```python
from build123d import *

# Parameters (mm, degrees)
BOSS_EXTRUDE1_DEPTH = 3.6
BOSS_EXTRUDE2_DEPTH = 1.5
CUT_EXTRUDE1_DEPTH  = 3.6
BOSS_EXTRUDE5_DEPTH = 3.6
CHAMFER1_SIZE       = 3.6
CHAMFER1_SIZE_2     = 0.062838234
FILLET3_R           = 1
FILLET4_R           = 0.5


with BuildPart() as part:
    # Sketch1 → Boss-Extrude1 (new body)
    with BuildSketch(Plane(origin=(0, 0, 0), x_dir=(1, 0, 0), z_dir=(0, 1, 0))):
        with BuildLine():
            Line((6, 0), (26.9, 0))
            ThreePointArc((26.9, 0), (31.142640687, 1.757359313), (32.9, 6))
            Line((32.9, 6), (32.9, 17.9))
            ThreePointArc((32.9, 17.9), (31.142640687, 22.142640687), (26.9, 23.9))
            Line((26.9, 23.9), (6, 23.9))
            ThreePointArc((6, 23.9), (1.757359313, 22.142640687), (0, 17.9))
            Line((0, 17.9), (0, 6))
            ThreePointArc((0, 6), (1.757359313, 1.757359313), (6, 0))
        make_face()
    extrude(amount=BOSS_EXTRUDE1_DEPTH)

    # Sketch2 → Boss-Extrude2 (add)
    with BuildSketch(Plane(origin=(0, 3.6, 0), x_dir=(1, 0, 0), z_dir=(0, 1, 0))):
        with BuildLine():
            Line((4.75, 25.15), (28.15, 25.15))
            ThreePointArc((28.15, 25.15), (33.099747468, 23.099747468), (35.15, 18.15))
            Line((35.15, 18.15), (35.15, 4.75))
            ThreePointArc((35.15, 4.75), (33.099747468, -0.199747468), (28.15, -2.25))
            Line((28.15, -2.25), (4.75, -2.25))
            ThreePointArc((4.75, -2.25), (-0.199747468, -0.199747468), (-2.25, 4.75))
            Line((-2.25, 4.75), (-2.25, 18.15))
            ThreePointArc((-2.25, 18.15), (-0.199747468, 23.099747468), (4.75, 25.15))
        make_face()
    extrude(amount=BOSS_EXTRUDE2_DEPTH)

    # Sketch3 → Cut-Extrude1 (cut)
    with BuildSketch(Plane.XZ):
        with BuildLine():
            Line((25.7, -22.7), (7.2, -22.7))
            ThreePointArc((7.2, -22.7), (2.957359313, -20.942640687), (1.2, -16.7))
            Line((1.2, -16.7), (1.2, -7.2))
            ThreePointArc((1.2, -7.2), (2.957359313, -2.957359313), (7.2, -1.2))
            Line((7.2, -1.2), (25.7, -1.2))
            ThreePointArc((25.7, -1.2), (29.942640687, -2.957359313), (31.7, -7.2))
            Line((31.7, -7.2), (31.7, -16.7))
            ThreePointArc((31.7, -16.7), (29.942640687, -20.942640687), (25.7, -22.7))
        make_face()
    extrude(amount=-CUT_EXTRUDE1_DEPTH, mode=Mode.SUBTRACT)

    # Sketch5 → Boss-Extrude5 (add)
    with BuildSketch(Plane.XZ.offset(-3.6)):
        with BuildLine():
            Line((7.2, -1.2), (8.4, -1.2))
            Line((8.4, -1.2), (8.4, -6.2))
            ThreePointArc((8.4, -6.2), (8.692893219, -6.907106781), (9.4, -7.2))
            Line((9.4, -7.2), (23.5, -7.2))
            ThreePointArc((23.5, -7.2), (24.207106781, -6.907106781), (24.5, -6.2))
            Line((24.5, -6.2), (24.5, -1.2))
            Line((24.5, -1.2), (25.7, -1.2))
            Line((25.7, -1.2), (25.7, -6.2))
            ThreePointArc((25.7, -6.2), (25.992893219, -6.907106781), (26.7, -7.2))
            Line((26.7, -7.2), (31.7, -7.2))
            Line((31.7, -7.2), (31.7, -8.4))
            Line((31.7, -8.4), (26.7, -8.4))
            ThreePointArc((26.7, -8.4), (25.992893219, -8.692893219), (25.7, -9.4))
            Line((25.7, -9.4), (25.7, -14.5))
            ThreePointArc((25.7, -14.5), (25.992893219, -15.207106781), (26.7, -15.5))
            Line((26.7, -15.5), (31.7, -15.5))
            Line((31.7, -15.5), (31.7, -16.7))
            Line((31.7, -16.7), (26.7, -16.7))
            ThreePointArc((26.7, -16.7), (25.992893219, -16.992893219), (25.7, -17.7))
            Line((25.7, -17.7), (25.7, -22.7))
            Line((25.7, -22.7), (24.5, -22.7))
            Line((24.5, -22.7), (24.5, -17.7))
            ThreePointArc((24.5, -17.7), (24.207106781, -16.992893219), (23.5, -16.7))
            Line((23.5, -16.7), (9.4, -16.7))
            ThreePointArc((9.4, -16.7), (8.692893219, -16.992893219), (8.4, -17.7))
            Line((8.4, -17.7), (8.4, -22.7))
            Line((8.4, -22.7), (7.2, -22.7))
            Line((7.2, -22.7), (7.2, -17.7))
            ThreePointArc((7.2, -17.7), (6.907106781, -16.992893219), (6.2, -16.7))
            Line((6.2, -16.7), (1.2, -16.7))
            Line((1.2, -16.7), (1.2, -15.5))
            Line((1.2, -15.5), (6.2, -15.5))
            ThreePointArc((6.2, -15.5), (6.907106781, -15.207106781), (7.2, -14.5))
            Line((7.2, -14.5), (7.2, -9.4))
            ThreePointArc((7.2, -9.4), (6.907106781, -8.692893219), (6.2, -8.4))
            Line((6.2, -8.4), (1.2, -8.4))
            Line((1.2, -8.4), (1.2, -7.2))
            Line((1.2, -7.2), (6.2, -7.2))
            ThreePointArc((6.2, -7.2), (6.907106781, -6.907106781), (7.2, -6.2))
            Line((7.2, -6.2), (7.2, -1.2))
        make_face()
        with BuildLine():
            Line((9.4, -8.4), (23.5, -8.4))
            ThreePointArc((23.5, -8.4), (24.207106781, -8.692893219), (24.5, -9.4))
            Line((24.5, -9.4), (24.5, -14.5))
            ThreePointArc((24.5, -14.5), (24.207106781, -15.207106781), (23.5, -15.5))
            Line((23.5, -15.5), (9.4, -15.5))
            ThreePointArc((9.4, -15.5), (8.692893219, -15.207106781), (8.4, -14.5))
            Line((8.4, -14.5), (8.4, -9.4))
            ThreePointArc((8.4, -9.4), (8.692893219, -8.692893219), (9.4, -8.4))
        make_face(mode=Mode.SUBTRACT)
    extrude(amount=BOSS_EXTRUDE5_DEPTH)

    # Chamfer1
    # the kernel refuses this chamfer: 3.6, 0.062838234 mm, written as the material it takes off along each edge
    with BuildSketch(Plane(origin=(0, 0, -17.9), x_dir=(-0.0006712501823120534, 0.9999997747115711, 0), z_dir=(0, 0, 1))) as chamfer1_piece_1_section:
        Polygon((CHAMFER1_SIZE * 0.999999774712, -CHAMFER1_SIZE * 0.000671250182312), (-CHAMFER1_SIZE_2 * 0.000671250179552, -CHAMFER1_SIZE_2 * 0.999999770599), (0, 0), align=None)
    chamfer1_piece_1 = extrude(amount=11.9, mode=Mode.PRIVATE)
    chamfer1_piece_1 = split(chamfer1_piece_1, bisect_by=Plane(origin=(-0.01902042, 3.6, -11.95), z_dir=(0, -1, 0)), keep=Keep.TOP, mode=Mode.PRIVATE)
    add(chamfer1_piece_1, mode=Mode.SUBTRACT)
    with BuildSketch(Plane(origin=(6, 0, -6), x_dir=(-1, 0, 0), z_dir=(0, 0, -1))) as chamfer1_piece_2_section:
        Polygon((6, CHAMFER1_SIZE), (6 - CHAMFER1_SIZE_2 * 0.999999995888, 0), (6, 0), align=None)
    chamfer1_piece_2 = revolve(axis=Axis((6, 0, -6), (0, 1, 0)), revolution_arc=90, mode=Mode.PRIVATE)
    chamfer1_piece_2 = split(chamfer1_piece_2, bisect_by=Plane(origin=(1.769655981, 3.6, -1.769655981), z_dir=(0, -1, 0)), keep=Keep.TOP, mode=Mode.PRIVATE)
    add(chamfer1_piece_2, mode=Mode.SUBTRACT)
    with BuildSketch(Plane(origin=(6, 0, -17.9), x_dir=(0, 0, -1), z_dir=(1, 0, 0))) as chamfer1_piece_3_section:
        Polygon((6, CHAMFER1_SIZE), (6 - CHAMFER1_SIZE_2 * 0.999999995888, 0), (6, 0), align=None)
    chamfer1_piece_3 = revolve(axis=Axis((6, 0, -17.9), (0, 1, 0)), revolution_arc=90, mode=Mode.PRIVATE)
    chamfer1_piece_3 = split(chamfer1_piece_3, bisect_by=Plane(origin=(1.769655981, 3.6, -22.130344019), z_dir=(0, -1, 0)), keep=Keep.TOP, mode=Mode.PRIVATE)
    add(chamfer1_piece_3, mode=Mode.SUBTRACT)
    with BuildSketch(Plane(origin=(6, 0, 0), x_dir=(0, 0.9999997747115711, 0.0006712501823120534), z_dir=(1, 0, 0))) as chamfer1_piece_4_section:
        Polygon((CHAMFER1_SIZE * 0.999999774712, -CHAMFER1_SIZE * 0.000671250182312), (-CHAMFER1_SIZE_2 * 0.000671250179552, -CHAMFER1_SIZE_2 * 0.999999770599), (0, 0), align=None)
    chamfer1_piece_4 = extrude(amount=20.9, mode=Mode.PRIVATE)
    chamfer1_piece_4 = split(chamfer1_piece_4, bisect_by=Plane(origin=(16.45, 3.6, 0.01902042), z_dir=(0, -1, 0)), keep=Keep.TOP, mode=Mode.PRIVATE)
    add(chamfer1_piece_4, mode=Mode.SUBTRACT)
    with BuildSketch(Plane(origin=(26.9, 0, -23.9), x_dir=(0, 0.9999997747115711, -0.0006712501823119971), z_dir=(-1, 0, 0))) as chamfer1_piece_5_section:
        Polygon((CHAMFER1_SIZE * 0.999999774712, -CHAMFER1_SIZE * 0.000671250182312), (-CHAMFER1_SIZE_2 * 0.000671250179552, -CHAMFER1_SIZE_2 * 0.999999770599), (0, 0), align=None)
    chamfer1_piece_5 = extrude(amount=20.9, mode=Mode.PRIVATE)
    chamfer1_piece_5 = split(chamfer1_piece_5, bisect_by=Plane(origin=(16.45, 3.6, -23.91902042), z_dir=(0, -1, 0)), keep=Keep.TOP, mode=Mode.PRIVATE)
    add(chamfer1_piece_5, mode=Mode.SUBTRACT)
    with BuildSketch(Plane(origin=(26.9, 0, -6), x_dir=(0, 0, 1), z_dir=(-1, 0, 0))) as chamfer1_piece_6_section:
        Polygon((6, CHAMFER1_SIZE), (6 - CHAMFER1_SIZE_2 * 0.999999995888, 0), (6, 0), align=None)
    chamfer1_piece_6 = revolve(axis=Axis((26.9, 0, -6), (0, 1, 0)), revolution_arc=90, mode=Mode.PRIVATE)
    chamfer1_piece_6 = split(chamfer1_piece_6, bisect_by=Plane(origin=(31.130344019, 3.6, -1.769655981), z_dir=(0, -1, 0)), keep=Keep.TOP, mode=Mode.PRIVATE)
    add(chamfer1_piece_6, mode=Mode.SUBTRACT)
    with BuildSketch(Plane(origin=(26.9, 0, -17.9), x_dir=(1, 0, 0), z_dir=(0, 0, 1))) as chamfer1_piece_7_section:
        Polygon((6, CHAMFER1_SIZE), (6 - CHAMFER1_SIZE_2 * 0.999999995888, 0), (6, 0), align=None)
    chamfer1_piece_7 = revolve(axis=Axis((26.9, 0, -17.9), (0, 1, 0)), revolution_arc=90, mode=Mode.PRIVATE)
    chamfer1_piece_7 = split(chamfer1_piece_7, bisect_by=Plane(origin=(31.130344019, 3.6, -22.130344019), z_dir=(0, -1, 0)), keep=Keep.TOP, mode=Mode.PRIVATE)
    add(chamfer1_piece_7, mode=Mode.SUBTRACT)
    with BuildSketch(Plane(origin=(32.9, 0, -6), x_dir=(0.000671250182312946, 0.9999997747115711, 0), z_dir=(0, 0, -1))) as chamfer1_piece_8_section:
        Polygon((CHAMFER1_SIZE * 0.999999774712, -CHAMFER1_SIZE * 0.000671250182313), (-CHAMFER1_SIZE_2 * 0.000671250179553, -CHAMFER1_SIZE_2 * 0.999999770599), (0, 0), align=None)
    chamfer1_piece_8 = extrude(amount=11.9, mode=Mode.PRIVATE)
    chamfer1_piece_8 = split(chamfer1_piece_8, bisect_by=Plane(origin=(32.91902042, 3.6, -11.95), z_dir=(0, -1, 0)), keep=Keep.TOP, mode=Mode.PRIVATE)
    add(chamfer1_piece_8, mode=Mode.SUBTRACT)

    # Fillet3
    fillet3_edges = [part.edges().sort_by_distance(p)[0] for p in [
        (1.2, 1.8, -8.4),
        (1.2, 1.8, -15.5),
        (8.4, 1.8, -22.7),
        (24.5, 1.8, -22.7),
        (31.7, 1.8, -15.5),
        (31.7, 1.8, -8.4),
        (24.5, 1.8, -1.2),
        (8.4, 1.8, -1.2),
        (7.2, 1.8, -22.7),
        (1.2, 1.8, -16.7),
        (1.2, 1.8, -7.2),
        (7.2, 1.8, -1.2),
        (25.7, 1.8, -1.2),
        (31.7, 1.8, -7.2),
        (31.7, 1.8, -16.7),
        (25.7, 1.8, -22.7),
    ]]
    fillet(fillet3_edges, radius=FILLET3_R)

    # Fillet4
    fillet4_edges = [part.edges().sort_by_distance(p)[0] for p in [
        (-0.199747468, 5.1, 0.199747468),
        (16.45, 5.1, 2.25),
        (33.099747468, 5.1, 0.199747468),
        (35.15, 5.1, -11.45),
        (33.099747468, 5.1, -23.099747468),
        (16.45, 5.1, -25.15),
        (-0.199747468, 5.1, -23.099747468),
        (-2.25, 5.1, -11.45),
    ]]
    fillet(fillet4_edges, radius=FILLET4_R)


solid = part.part
```
Geometry check sheet. Reference: the model listing, model coordinates, mm. A direction names the side the tool comes from. Round coordinates to 2 decimals unless told otherwise and drop trailing zeros. Loops run counter-clockwise (first coordinate to the right, second up) from the corner with the lowest first, then second, coordinate; pieces in that order, holes last. Notation, with made-up numbers: (73, -1.5) - (131, -1.5) arc R30 ccw to (131, 35.5) - close; hole circle Ø9 at (-32.75, 84.5). An arc over 180 degrees is marked (long way). Use a Markdown table: item, result.
Q1. Material ranges on line 1 (X direction, y = 0.3, z = -14.5); line 2 (Z direction, x = 27, y = 2.4); line 3 (X direction, y = 2.5, z = -8.75), recorded low to high.
Solutions:
| item | result |
|---|---|
| line 1 | x = 0.06 to 1.2, 7.2 to 8.4, 24.5 to 25.7, 31.7 to 32.84 |
| line 2 | z = -23.88 to -22.56, -16.7 to -15.5, -8.4 to -7.2, -1.34 to -0.02 |
| line 3 | x = 0.02 to 1.44, 6.96 to 8.64, 24.26 to 25.94, 31.46 to 32.88 |
Q2. Go/stop test with flat-tipped pins: P1, Ø3, axis at x = 17, y = 2, coming from the -Z side; P2, Ø3, axis at x = 27.5, z = -19, coming from the -Y side; P3, Ø1.8, axis at x = 3.5, y = 1.5, coming from the -Z side; P4, Ø6.5, axis at x = 5.5, z = -5, coming from the -Y side. Record where each tip stops, or that it passes through.
Solutions:
| item | result |
|---|---|
| P1 | stops at z = -23.9 |
| P2 | stops at y = 3.6 |
| P3 | stops at z = -23.65 |
| P4 | stops at y = 0 |
Q3. Cross-section at B-B on z = -10. Record the cut outline in (x, y).
Solutions:
| item | result |
|---|---|
| outline | (-2.25, 3.6) - (0, 3.6) - (0.06, 0) - (1.2, 0) - (1.2, 3.6) - (7.2, 3.6) - (7.2, 0) - (8.4, 0) - (8.4, 3.6) - (24.5, 3.6) - (24.5, 0) - (25.7, 0) - (25.7, 3.6) - (31.7, 3.6) - (31.7, 0) - (32.84, 0) - (32.9, 3.6) - (35.15, 3.6) - (35.15, 4.6) arc R0.5 ccw to (34.65, 5.1) - (-1.75, 5.1) arc R0.5 ccw to (-2.25, 4.6) - close |
Q4. Draft check along X on faces 3 (the flat face through (17, 5.1, -12)), 4 (the flat face through (35.15, 4, -12)), 5 (the flat face through (16, 2, -8.4)). Enter one of: released by +X, released by -X, zero draft, split by the parting line, or undercut.
Solutions:
| item | result |
|---|---|
| face 3 | zero draft |
| face 4 | released by +X |
| face 5 | undercut |
Q5. Cross-section at A-A on x = 14. Record the cut outline in (y, z), plus the area to 3 significant figures.
Solutions:
| item | result |
|---|---|
| outline | (0, -23.84) - (3.6, -23.9) - (3.6, -25.15) - (4.6, -25.15) arc R0.5 ccw to (5.1, -24.65) - (5.1, 1.75) arc R0.5 ccw to (4.6, 2.25) - (3.6, 2.25) - (3.6, 0) - (0, -0.06) - (0, -1.2) - (3.6, -1.2) - (3.6, -7.2) - (0, -7.2) - (0, -8.4) - (3.6, -8.4) - (3.6, -15.5) - (0, -15.5) - (0, -16.7) - (3.6, -16.7) - (3.6, -22.7) - (0, -22.7) - close |
| area | 58.0 mm2 |
Q6. Cross-section at D-D on y = 0.5. State how many separate pieces and enclosed holes the cut face has, plus the area to 3 significant figures.
Solutions:
| item | result |
|---|---|
| separate pieces | 1 |
| enclosed holes | 9 |
| area | 251 mm2 |
Q7. Access from +Z, -Z, +X, -X, +Y, -Y to the whole of each face (thin tool, end or side, straight path). Record for faces 1 (the cylindrical face through (33, 4.1, -23.2)), 2 (the flat face through (7.2, 2, -4)).
Solutions:
| item | result |
|---|---|
| face 1 | -Z, +X, +Y, -Y |
| face 2 | -Y |
Q8. Cross-section at C-C on y = 4.15. Record the cut outline in (x, z).
Solutions:
| item | result |
|---|---|
| outline | (-2.25, -18.15) arc R7 ccw to (4.75, -25.15) - (28.15, -25.15) arc R7 ccw to (35.15, -18.15) - (35.15, -4.75) arc R7 ccw to (28.15, 2.25) - (4.75, 2.25) arc R7 ccw to (-2.25, -4.75) - close |
